The listing builds one solid part. Answer for the finished solid, in the listing's coordinates (mm). Round coordinates to 2 decimals unless told otherwise and drop trailing zeros. Write each loop counter-clockwise with the first axis right and the second up, starting at its lowest first coordinate (ties: lowest second). Pieces come first, ordered by that corner, then holes.
(1) This flat-tipped pin is pushed along its axis until it touches: pin 1 Ø2.5 at (x, y) = (-15, 10) entering from +Z (3 decimals). Where does it stop, or does it pass through?
(2) A cutting plane is placed at B-B, the plane z = 2.45. Give the number of separate pieces and of enclosed holes in the cut face, and give its area (3 significant figures).
(3) A cutting plane is placed at A-A, the plane y = -30. Give the vertices of the cut face in (x, z), and give its area (3 significant figures).
(4) Find the intervals of material crossed by probe 1 along X at (y, z) = (-10, 2.1); probe 2 along Y at (x, z) = (15, 1.55); probe 3 along Y at (x, z) = (14, 0.55), in increasing order.
from build123d import *

# Parameters (mm, degrees)
SKETCH_1_W          = 40
SKETCH_1_H          = 72
EXTRUDE_1_DEPTH     = 3
SKETCH_2_R          = 1.5
CUT_EXTRUDE_1_DEPTH = 3
FILLET_1_R          = 5


with BuildPart() as part:
    # 草图1 → 凸台-拉伸1 (new body)
    with BuildSketch(Plane.XY):
        Rectangle(SKETCH_1_W, SKETCH_1_H)
    extrude(amount=EXTRUDE_1_DEPTH)

    # 草图2 → 切除-拉伸1 (cut)
    with BuildSketch(Plane.XY.offset(3)):
        with Locations((-15, 30)):
            Circle(SKETCH_2_R)
        with Locations((-15, 10)):
            Circle(SKETCH_2_R)
        with Locations((15, 30)):
            Circle(SKETCH_2_R)
        with Locations((15, 10)):
            Circle(SKETCH_2_R)
        with Locations(Location((-15, -10, 0), (0, 0, 180))):
            Circle(SKETCH_2_R)
        with Locations(Location((15, -10, 0), (0, 0, 180))):
            Circle(SKETCH_2_R)
        with Locations(Location((15, -30, 0), (0, 0, 180))):
            Circle(SKETCH_2_R)
        with Locations(Location((-15, -30, 0), (0, 0, 180))):
            Circle(SKETCH_2_R)
    extrude(amount=-CUT_EXTRUDE_1_DEPTH, mode=Mode.SUBTRACT)

    # 圆角1
    fillet_1_edges = [part.edges().sort_by_distance(p)[0] for p in [
        (20, -36, 1.5),
        (-20, -36, 1.5),
        (-20, 36, 1.5),
        (20, 36, 1.5),
    ]]
    fillet(fillet_1_edges, radius=FILLET_1_R)


solid = part.part
Solutions:
1. pin 1: passes through
2. separate pieces: 1
2. enclosed holes: 8
2. area: 2,800 mm2
3. outline: (-20, 0) - (-16.5, 0) - (-16.5, 3) - (-20, 3) - close; (-13.5, 0) - (13.5, 0) - (13.5, 3) - (-13.5, 3) - close; (16.5, 0) - (20, 0) - (20, 3) - (16.5, 3) - close
3. area: 102 mm2
4. probe 1: x = -20 to -16.5, -13.5 to 13.5, 16.5 to 20
4. probe 2: y = -36 to -31.5, -28.5 to -11.5, -8.5 to 8.5, 11.5 to 28.5, 31.5 to 36
4. probe 3: y = -36 to -31.12, -28.88 to -11.12, -8.88 to 8.88, 11.12 to 28.88, 31.12 to 36
